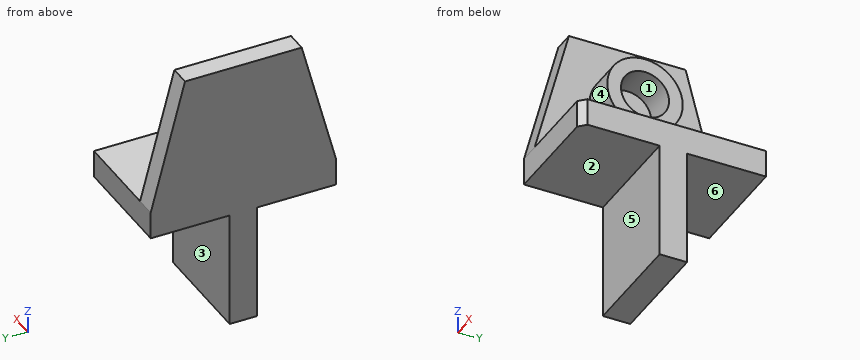
from build123d import *

# Parameters (mm, degrees)
F1_DEPTH = 32
F3_DEPTH = 6
F4_R     = 11
F4_R_2   = 7
F5_DEPTH = 10
F6_SIZE  = 2


with BuildPart() as f1:
    # F0 (on Right) → F1 (new body)
    with BuildSketch(Plane.YZ):
        Polygon((27, 0), (-27, 0), (-27, -8), (-4, -8), (-4, -42), (4, -42), (4, -8), (27, -8), align=None)
    extrude(amount=-F1_DEPTH)

    # F2 (on face) → F3 (join)
    with BuildSketch(Plane(origin=(-32, 0, 0), x_dir=(0, -1, 0), z_dir=(-1, 0, 0))):
        Polygon((-27, 0), (27, 0), (17, 38), (-17, 38), align=None)
    extrude(amount=-F3_DEPTH)

    # F4 (on face) → F5 (join)
    with BuildSketch(Plane.YZ.offset(-26)):
        with Locations((0, 19)):
            Circle(F4_R)
        with Locations((0, 19)):
            Circle(F4_R_2, mode=Mode.SUBTRACT)
    extrude(amount=F5_DEPTH)

    # F6
    f6_edges = [f1.edges().sort_by_distance(p)[0] for p in [
        (0, -27, -4),
    ]]
    chamfer(f6_edges, length=F6_SIZE)


solid = f1.part
Work out the finished part from the listing and answer in its coordinate system (mm). Face numbers are marked on the shaded views. A direction names the side the tool comes from. Round coordinates to 2 decimals unless told otherwise and drop trailing zeros. Loops run counter-clockwise (first coordinate to the right, second up) from the corner with the lowest first, then second, coordinate; pieces in that order, holes last. Notation, with made-up numbers: (75.5, -21) - (132.5, -21) arc R17 ccw to (132.5, 5) - close; hole circle Ø9 at (52.25, 76). An arc over 180 degrees is marked (long way). Use one line per item in the form item = value. Start each with the question number.
(1) Find section B-B on x = -8. Determine the outline of the cut face in (y, z).
(2) Determine the mould class of the marked faces 1, 2 and 3 for opening direction Z: +Z half, -Z half, draft (parallel to the pull), parting line (faces both ways), or undercut.
(3) Find section A-A on x = -21.5. Determine the outline of the cut face in (y, z).
(4) Consider line 1 (Z direction, x = -23, y = 0); line 2 (Z direction, x = -9, y = -18.5); line 3 (Z direction, x = -23, y = 7.5). Determine where each line is inside the solid, lowest interval first.
(5) Find section D-D on z = 19. Determine the outline of the cut face in (x, y), and give its area (3 significant figures).
(6) Which of the six approach directions +Z, -Z, +X, -X, +Y, -Y give full straight-line access (tool end or side, diameter ignored) to the marked faces 4, 5 and 6?
(7) Find section C-C on y = 6. Determine the outline of the cut face in (x, z).
(8) Flat-ended cylindrical pins translate along their axes: P1, Ø3, axis at x = -7, z = -24, coming from the -Y side; P2, Ø4, axis at x = -5, y = -8.5, coming from the +Z side; P3, Ø1.5, axis at y = 16, z = 15.5, coming from the +X side. Find the tip coordinate at first contact, or state that the pin passes through.
Answer list:
q1.outline = (-27, -8) - (-4, -8) - (-4, -42) - (4, -42) - (4, -8) - (27, -8) - (27, 0) - (-27, 0) - close
q2.face_1 = undercut
q2.face_2 = -Z half
q2.face_3 = draft
q3.outline = (-27, -8) - (-4, -8) - (-4, -42) - (4, -42) - (4, -8) - (27, -8) - (27, 0) - (-27, 0) - close; circle Ø22 at (0, 19); hole circle Ø14 at (0, 19)
q4.line_1 = -42 to 0, 8 to 12, 26 to 30
q4.line_2 = -8 to 0
q4.line_3 = -8 to 0, 10.95 to 27.05
q5.outline = (-32, -22) - (-26, -22) - (-26, -11) - (-16, -11) - (-16, -7) - (-26, -7) - (-26, 7) - (-16, 7) - (-16, 11) - (-26, 11) - (-26, 22) - (-32, 22) - close
q5.area = 344 mm^2
q6.face_4 = +X
q6.face_5 = -Z, +X, -X, -Y
q6.face_6 = -Z, +X, -X, +Y
q7.outline = (-32, -8) - (0, -8) - (0, 0) - (-26, 0) - (-26, 9.78) - (-16, 9.78) - (-16, 15.39) - (-26, 15.39) - (-26, 22.61) - (-16, 22.61) - (-16, 28.22) - (-26, 28.22) - (-26, 38) - (-32, 38) - close
q8.P1 = -4
q8.P2 = 0
q8.P3 = -26
